Input: dimensioned drawing with shaded views. Units: mm. Origin: part minimum x, y, z. Coordinates: 2 decimals unless noted, no trailing zeros. Order: outer loops, then holes, each group sorted by start corner. A loop starts at its lowest first (then second) coordinate and runs counter-clockwise, first axis right, second up.
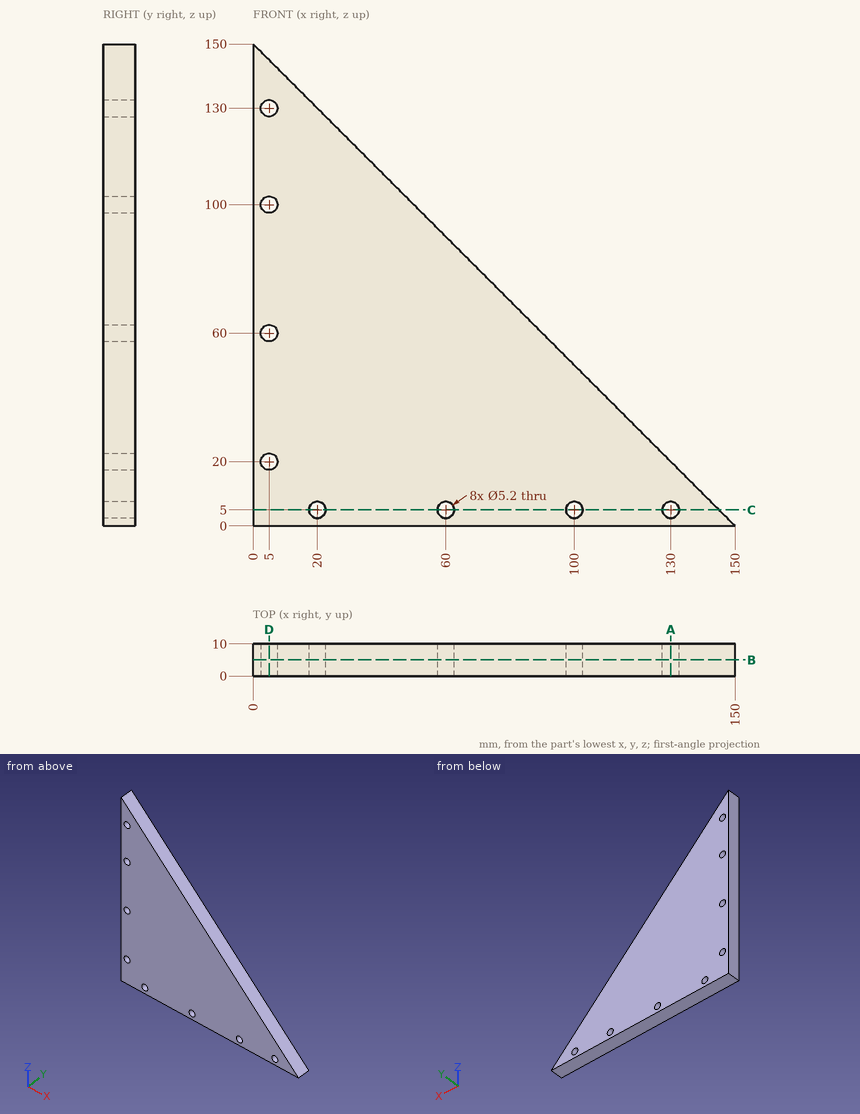
1. Pin query (flat end, axial travel): P1, Ø1, axis at x = 126, y = 6, coming from the +Z side; P2, Ø3, axis at x = 60, z = 5, coming from the +Y side. Return the tip coordinate at first contact, or that it passes through.
Findings:
P1: stops at z = 24.5
P2: passes through
2. Section query D-D on x = 5. Return loops of the section in (y, z), plus the area to 3 significant figures.
Findings:
outline: (0, 0) - (10, 0) - (10, 17.4) - (0, 17.4) - close; (0, 22.6) - (10, 22.6) - (10, 57.4) - (0, 57.4) - close; (0, 62.6) - (10, 62.6) - (10, 97.4) - (0, 97.4) - close; (0, 102.6) - (10, 102.6) - (10, 127.4) - (0, 127.4) - close; (0, 132.6) - (10, 132.6) - (10, 145) - (0, 145) - close
area: 1,240 mm2
3. Section query C-C on z = 5. Return loops of the section in (x, y), plus the area to 3 significant figures.
Findings:
outline: (0, 0) - (17.4, 0) - (17.4, 10) - (0, 10) - close; (22.6, 0) - (57.4, 0) - (57.4, 10) - (22.6, 10) - close; (62.6, 0) - (97.4, 0) - (97.4, 10) - (62.6, 10) - close; (102.6, 0) - (127.4, 0) - (127.4, 10) - (102.6, 10) - close; (132.6, 0) - (145, 0) - (145, 10) - (132.6, 10) - close
area: 1,240 mm2
4. Ray query, line 1 (X direction, y = 6.5, z = 5); line 2 (X direction, y = 7.5, z = 129.5). Return the intervals inside material, ascending.
Findings:
line 1: x = 0 to 17.4, 22.6 to 57.4, 62.6 to 97.4, 102.6 to 127.4, 132.6 to 145
line 2: x = 0 to 2.45, 7.55 to 20.5
5. Section query B-B on y = 5. Count the separate pieces of the cut face and the enclosed holes in it, plus the area to 3 significant figures.
Findings:
separate pieces: 1
enclosed holes: 8
area: 11,100 mm2
6. Section query A-A on x = 130. Return loops of the section in (y, z).
Findings:
outline: (0, 0) - (10, 0) - (10, 2.4) - (0, 2.4) - close; (0, 7.6) - (10, 7.6) - (10, 20) - (0, 20) - close
